Autodesk Inventor part; units mm, degrees
ref_plane "YZ Plane" through (0, 0, 0) normal (1, 0, 0) x (0, 1, 0)
ref_plane "XZ Plane" through (0, 0, 0) normal (0, 1, 0) x (-1, 0, 0)
ref_plane "XY Plane" through (0, 0, 0) normal (0, 0, 1) x (1, 0, 0)
sketch "Sketch1" plane through (0, 0, 0) normal (0, 1, 0) x (-1, 0, 0)
  line L0 (0, 0) -> (-60, 0)
  line L1 (-60, 0) -> (-60, 10)
  line L2 (-60, 10) -> (0, 10)
  line L3 (0, 10) -> (0, 0)
  dimension "d0" = 60
  dimension "d1" = 10
extrude "Extrusion1" add sketch "Sketch1" along normal blind 2
sketch "Sketch2" plane through (0, 2, 0) normal (0, 1, 0) x (1, 0, 0)
  line L0 (0, 0) -> (0, -10)
  line L1 (0, 0) -> (10, 0)
  line L2 (10, 0) -> (10, -9.6)
  line L3 (10, -9.6) -> (0, -9.6)
  line L4 (0, -9.6) -> (0, 0)
  line L5 (60, -10) -> (60, 0)
  line L6 (60, 0) -> (50, 0)
  line L7 (50, 0) -> (50, -9.6)
  line L8 (50, -9.6) -> (60, -9.6)
  line L9 (60, -9.6) -> (60, 0)
  dimension "d4" = 10
  dimension "d5" = 9.6
  dimension "d6" = 10
  dimension "d7" = 9.6
extrude "Extrusion2" add sketch "Sketch2" along normal blind 36.85
sketch "Sketch3" plane through (0, 2, 9.6) normal (0, 0, 1) x (1, 0, 0)
  line L0 (0, -2) -> (0, 36.85)
  line L1 (10, 0) -> (10, 36.85)
  line L2 (0, 36.85) -> (10, 36.85)
  line L3 (10, 36.85) -> (10, 31.85)
  line L4 (10, 31.85) -> (0, 31.85)
  line L5 (0, 31.85) -> (0, 36.85)
  line L6 (50, 0) -> (50, 36.85)
  line L7 (60, -2) -> (60, 36.85)
  line L8 (50, 36.85) -> (60, 36.85)
  line L9 (60, 36.85) -> (60, 31.85)
  line L10 (60, 31.85) -> (50, 31.85)
  line L11 (50, 31.85) -> (50, 36.85)
  point P0 (0, 31.85)
  dimension "d10" = 5
  dimension "d11" = 5
extrude "Extrusion3" add sketch "Sketch3" along normal blind 2
sketch "Sketch4" plane through (60, 0, 0) normal (0, 0, -1) x (-1, 0, 0)
  line L0 (0, 0) -> (0, 38.85)
  line L1 (10, 2) -> (10, 38.85)
  line L2 (0, 38.85) -> (10, 38.85)
  line L3 (10, 38.85) -> (10, 33.85)
  line L4 (10, 33.85) -> (0, 33.85)
  line L5 (0, 33.85) -> (0, 38.85)
  line L6 (50, 2) -> (50, 38.85)
  line L7 (60, 0) -> (60, 38.85)
  line L8 (50, 38.85) -> (60, 38.85)
  line L9 (60, 38.85) -> (60, 33.85)
  line L10 (60, 33.85) -> (50, 33.85)
  line L11 (50, 33.85) -> (50, 38.85)
  point P0 (0, 33.85)
  dimension "d14" = 5
  dimension "d15" = 5
extrude "Extrusion4" add sketch "Sketch4" along normal blind 2
sketch "Sketch5" plane through (0, 0, 0) normal (-1, 0, 0) x (0, 0, 1)
  line L0 (-2, 38.85) -> (11.6, 38.85)
  circle A0 centre (4.8, 38.85) radius 4.75
  point P0 (0, 0)
  dimension "d18" = 9.5
extrude "Extrusion5" cut sketch "Sketch5" against normal through all
fillet "Fillet1" radius 2 8 edges at (55, 33.85, 0) (55, 33.85, 9.6) (55, 33.85, 11.6) (55, 33.85, -2) (5, 33.85, 0) (5, 33.85, -2) (5, 33.85, 9.6) (5, 33.85, 11.6)
fillet "Fillet2" radius 2 2 edges at (30, 2, 10) (30, 2, 0)
properties part number "dg_mount"
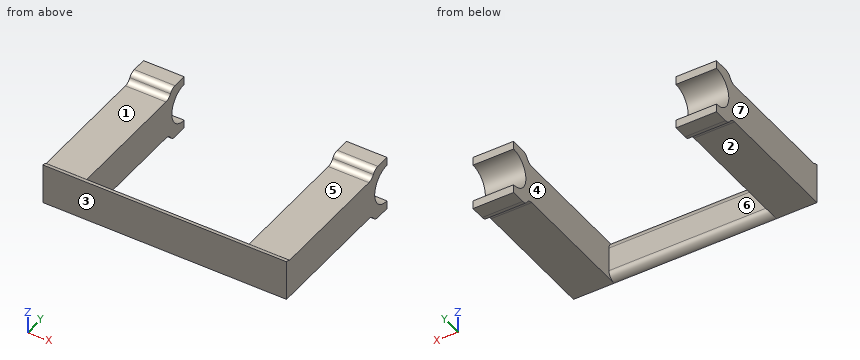
The listing builds one solid part. Answer for the finished solid, in the listing's coordinates (mm). Face numbers are marked on the shaded views. A direction names the side the tool comes from. Coordinates: 2 decimals unless noted, no trailing zeros. Write each loop counter-clockwise with the first axis right and the second up, starting at its lowest first coordinate (ties: lowest second). Pieces come first, ordered by that corner, then holes. Notation, with made-up numbers: (12.25, -8) - (68.25, -8) arc R31 ccw to (68.25, 22) - close; hole circle Ø4 at (25, -4.5). An arc over 180 degrees is marked (long way). Put each result on its own line as item: value.
1. A tool of negligible diameter and unlimited length cuts with its end or side. For the marked faces 1, 2 and 3, from which of +Z, -Z, +X, -X, +Y, -Y can it reach the whole face along a straight path? Write none if from no direction.
Answer sheet:
face 1: +Z, +X, -X
face 2: -Z, +X, -X, -Y
face 3: +Z, -Z, +X, -X, -Y
2. Determine the mould class of the marked faces 4, 5, 6 and 7 for opening direction X: pulls with the +X half, pulls with the -X half, needs draft (parallel to the pull), parting line crosses it, or undercut.
Answer sheet:
face 4: undercut
face 5: needs draft
face 6: undercut
face 7: pulls with the -X half
3. Find the intervals of material crossed by line 1 along X through (y, z) = (14.5, 7.75); line 2 along Z through (x, y) = (53.5, 11); line 3 along Y through (x, z) = (30, 4.5), in increasing order. Write a range as from..to.
Answer sheet:
line 1: x = 0..10, 50..60
line 2: z = 0..9.6
line 3: y = 0..2
4. The part is cut by section B-B on z = 4.8. Give the vertices of the cut face in (x, y).
Answer sheet:
outline: (0, 0) - (60, 0) - (60, 34.1) - (50, 34.1) - (50, 2) - (10, 2) - (10, 34.1) - (0, 34.1) - close
5. Flat-ended cylindrical pins translate along their axes: pin 1 Ø12 at (x, y) = (8.5, 14) entering from +Z; pin 2 Ø7 at (y, z) = (26.5, 4) entering from -X; pin 3 Ø2 at (x, z) = (36, 3.5) entering from +Y; pin 4 Ø1 at (x, z) = (9, 2.5) entering from +Y. Find the tip coordinate at first contact, or state that the pin passes through.
Answer sheet:
pin 1: stops at z = 9.6
pin 2: stops at x = 0
pin 3: stops at y = 2
pin 4: stops at y = 35.01
6. The part is cut by section A-A on y = 16.5. Give the vertices of the cut face in (x, z).
Answer sheet:
outline: (0, 0) - (10, 0) - (10, 9.6) - (0, 9.6) - close; (50, 0) - (60, 0) - (60, 9.6) - (50, 9.6) - close
